```python
from build123d import *

# Parameters (mm, degrees)
SKETCH1_W           = 48
SKETCH1_H           = 25
SKETCH1_R           = 1.55
SKETCH1_R_2         = 2.05
BOSS_EXTRUDE1_DEPTH = 6
FILLET1_R           = 3
FILLET2_R           = 3
FILLET3_R           = 3
FILLET4_R           = 3


with BuildPart() as part:
    # Sketch1 → Boss-Extrude1 (new body)
    with BuildSketch(Plane.XY):
        with Locations((-2.366412214, -1.965648855)):
            Rectangle(SKETCH1_W, SKETCH1_H)
        with Locations((-8.023266463, 3.691205395)):
            Circle(SKETCH1_R, mode=Mode.SUBTRACT)
        with Locations((-8.023266463, -7.622503104)):
            Circle(SKETCH1_R, mode=Mode.SUBTRACT)
        with Locations((3.290442036, -7.622503104)):
            Circle(SKETCH1_R, mode=Mode.SUBTRACT)
        with Locations((3.290442036, 3.691205395)):
            Circle(SKETCH1_R, mode=Mode.SUBTRACT)
        with Locations((-18.366412214, 6.034351145)):
            Circle(SKETCH1_R_2, mode=Mode.SUBTRACT)
        with Locations((13.633587786, 6.034351145)):
            Circle(SKETCH1_R_2, mode=Mode.SUBTRACT)
        with Locations((13.633587786, -9.965648855)):
            Circle(SKETCH1_R_2, mode=Mode.SUBTRACT)
        with Locations((-18.366412214, -9.965648855)):
            Circle(SKETCH1_R_2, mode=Mode.SUBTRACT)
    extrude(amount=BOSS_EXTRUDE1_DEPTH)

    # Fillet1
    fillet1_edges = [part.edges().sort_by_distance(p)[0] for p in [
        (21.633587786, -14.465648855, 3),
    ]]
    fillet(fillet1_edges, radius=FILLET1_R)

    # Fillet2
    fillet2_edges = [part.edges().sort_by_distance(p)[0] for p in [
        (-26.366412214, -14.465648855, 3),
    ]]
    fillet(fillet2_edges, radius=FILLET2_R)

    # Fillet3
    fillet3_edges = [part.edges().sort_by_distance(p)[0] for p in [
        (21.633587786, 10.534351145, 3),
    ]]
    fillet(fillet3_edges, radius=FILLET3_R)

    # Fillet4
    fillet4_edges = [part.edges().sort_by_distance(p)[0] for p in [
        (-26.366412214, 10.534351145, 3),
    ]]
    fillet(fillet4_edges, radius=FILLET4_R)


solid = part.part
```
Could you check a few things on this model? Use its own coordinates, in mm. Round coordinates to 2 decimals unless told otherwise and drop trailing zeros. Order: outer loops, then holes, each group sorted by start corner. A loop starts at its lowest first (then second) coordinate and runs counter-clockwise, first axis right, second up. Notation, with made-up numbers: M -9,35.5 L 17,35.5 A32 ccw 17,66.5 Z; hole C -10.75,-9 d2. An arc over 180 degrees is marked long. One line per question, with ' | ' between items. Start each with the question number.
(1) Thinking about a two-plate mould opening in Y: for faces 1 (the face through (12.007, -11.213, 2.958)), 2 (the face through (-3, -2, 6)), 3 (the face through (20.78, 9.63, 3.04)), 4 (the face through (12.007, 4.787, 2.958)), which applies, +Y half, -Y half, draft (parallel to the pull), parting line (faces both ways), or undercut?
(2) For P1, Ø5, axis at x = -8.02, y = -7.62, coming from the -Z side, with a flat end and sliding along its axis, tell me the tip position at first contact or that it passes through.
(3) Please list where these lines run through material, in increasing order: line 1 along X through (y, z) = (-9.75, 2.5); line 2 along X through (y, z) = (-7.75, 3.95); line 3 along Y through (x, z) = (-8, 3.4).
(4) Suppose I cut it at B-B on y = 7. List the corners of the cut face in (x, z) for me, then the cut area to 3 significant figures.
(5) Suppose I cut it at A-A on x = 15. List the corners of the cut face in (y, z) for me, then the cut area to 3 significant figures.
(6) Suppose I cut it at C-C on z = 2.2. Count the separate pieces of the cut face and the enclosed holes in it, then the cut area to 3 significant figures.
Geometry results:
1) face 1: undercut | face 2: draft | face 3: +Y half | face 4: undercut
2) P1: z = 0
3) line 1: -26.37 to -20.41, -16.33 to 11.59, 15.67 to 21.63 | line 2: -26.37 to -9.57, -6.48 to 1.75, 4.84 to 21.63 | line 3: -14.47 to -9.17, -6.07 to 2.14, 5.24 to 10.53
4) outline: M -26.37,0 L -20.17,0 L -20.17,6 L -26.37,6 Z; M -16.56,0 L 11.83,0 L 11.83,6 L -16.56,6 Z; M 15.44,0 L 21.63,0 L 21.63,6 L 15.44,6 Z | area: 245 mm²
5) outline: M -14.47,0 L -11.49,0 L -11.49,6 L -14.47,6 Z; M -8.44,0 L 4.51,0 L 4.51,6 L -8.44,6 Z; M 7.56,0 L 10.53,0 L 10.53,6 L 7.56,6 Z | area: 113 mm²
6) separate pieces: 1 | enclosed holes: 8 | area: 1,110 mm²
